from build123d import *


with BuildPart() as part:
    # Sketch1 → Revolve3 (revolve)
    with BuildSketch(Plane.XY, mode=Mode.PRIVATE) as revolve3_sk:
        with BuildLine():
            Line((0, 0), (1, 0))
            ThreePointArc((1, 0), (1.012509778, -1.000312842), (1.050031289, -2))
            Line((1.050031289, -2), (2.051315812, -2))
            ThreePointArc((2.051315812, -2), (2.012831064, -1.00032911), (2, 0))
            ThreePointArc((2, 0), (5.180088034, 6.896539681), (11.570458359, 11))
            Line((11.570458359, 11), (41, 11))
            Line((41, 11), (41, 13))
            Line((41, 13), (11.364514255, 13))
            ThreePointArc((11.364514255, 13), (3.709713219, 8.224384875), (0, 0))
        make_face()
    revolve(revolve3_sk.sketch.rotate(Axis((41, 13, 0), (0, -1, 0)), 270), axis=Axis((41, 13, 0), (0, -1, 0)))


solid = part.part
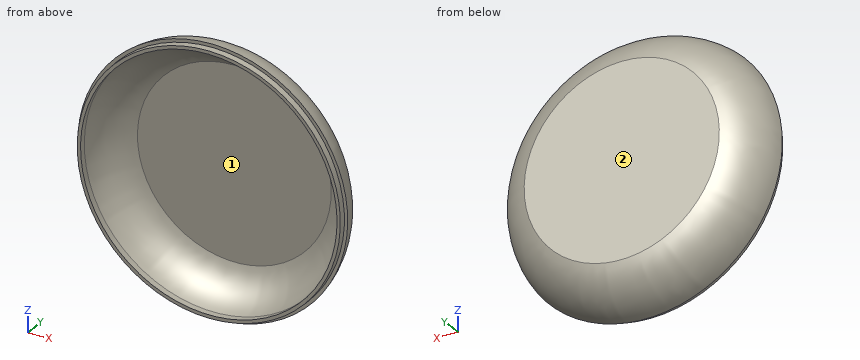
Check sheet for the modelled part. Datum: model origin and axes. Units: mm. Face numbers are marked on the shaded views. Round coordinates to 2 decimals unless told otherwise and drop trailing zeros. Loops run counter-clockwise (first coordinate to the right, second up) from the corner with the lowest first, then second, coordinate; pieces in that order, holes last. Notation, with made-up numbers: M -3,5 L 55,5 A21 cw 55,17 Z; hole C 71.5,80.5 d4. An arc over 180 degrees is marked long. One line per question, with ' | ' between items. Start each with the question number.
Item 1: Release check for a two-part mould opening along Z. For the marked faces 1 and 2 record: released by +Z, released by -Z, zero draft, split by the parting line, or undercut.
Item 2: Scan lines: probe 1 along Y at (x, z) = (28, -23); probe 2 along Z at (x, y) = (44.5, 10.5); probe 3 along X at (y, z) = (0.75, -17.5). Record each from-to range of solid material in increasing order.
Item 3: Gauge pin test, flat ends, axial feed: pin 1 Ø6 at (y, z) = (2.5, -13) entering from +X; pin 2 Ø2 at (y, z) = (9.5, -17.5) entering from -X; pin 3 Ø10 at (x, z) = (19, 13.5) entering from -Y. Record the tip position at first contact, or that the pin passes through.
Item 4: Section check B-B (y = 12). Record the boundary of the cut face in (x, z).
Item 5: Section check A-A (y = 4). Record the boundary of the cut face in (x, z).
Worked out:
1) face 1: undercut | face 2: zero draft
2) probe 1: 11 to 13 | probe 2: -34.64 to -30.64, 30.64 to 34.64 | probe 3: 4.05 to 6.3, 75.7 to 77.95
3) pin 1: x = 80.5 | pin 2: x = 8.23 | pin 3: y = 10.51
4) outline: C 41,0 d64.65
5) outline: C 41,0 d79.85; hole C 41,0 d75.5
